Geometry: final body of the model. Coordinates: model frame, mm. A direction names the side the tool comes from. Coordinates: 2 decimals unless noted, no trailing zeros. Order: outer loops, then holes, each group sorted by start corner. A loop starts at its lowest first (then second) coordinate and runs counter-clockwise, first axis right, second up. Notation, with made-up numbers: M -38,-14 L -23,-14 A24 ccw -23,9 Z; hole C 50,-23.5 d10. An arc over 180 degrees is marked long. Use CSV: the item, a comma, the result in double quotes. Start each with the question number.
Q1. Access query for faces 1 (the face through (0, 22.5, 0)), 2 (the face through (7.277, 22.246, -7.936)). Directions: +Z, -Z, +X, -X, +Y, -Y. A direction counts if a zero-diameter tool reaches every point of the face in a straight line with its end or side. Return the directions, or none.
Q2. Ray query, probe 1 along X at (y, z) = (7.5, 6.5); probe 2 along Z at (x, y) = (7.5, 8.75); probe 3 along Z at (x, y) = (-10.5, 20.5). Return the intervals inside material, ascending.
Q3. First-contact query: P1, Ø8, axis at x = 9, y = 4, coming from the +Z side; P2, Ø8, axis at x = 12.5, z = -5, coming from the +Y side; P3, Ø3, axis at x = -4.5, y = 6, coming from the -Z side; P4, Ø2, axis at x = -8.5, y = 6.5, coming from the +Z side. Flat tips, straight axial feed; report the tip coordinate or a pass-through.
Q4. Section query C-C, the plane y = 14. Output: boundary loops of the cut face in (x, z).
Q5. Section query A-A, the plane z = 0. Output: boundary loops of the cut face in (x, y).
Q6. Section query B-B, the plane y = 4.25. Output: boundary loops of the cut face in (x, z), and give its area (3 significant figures).
from build123d import *

# Parameters (mm, degrees)
SKETCH_1_R      = 17
EXTRUDE_1_DEPTH = 8
SKETCH_2_R      = 17
EXTRUDE_2_DEPTH = 14
EXTRUDE_2_TAPER = 24
SKETCH_4_R      = 10.766798406
EXTRUDE_3_DEPTH = 0.5


with BuildPart() as part:
    # 草图1 → 凸台-拉伸1 (new body)
    with BuildSketch(Plane(origin=(0, 0, 0), x_dir=(1, 0, 0), z_dir=(0, 1, 0))):
        with Locations(Location((0, 0, 0), (0, 0, 270))):
            Circle(SKETCH_1_R)
    extrude(amount=EXTRUDE_1_DEPTH)

    # 草图2 → 凸台-拉伸2 (add)
    with BuildSketch(Plane(origin=(0, 8, 0), x_dir=(1, 0, 0), z_dir=(0, 1, 0))):
        with Locations(Location((0, 0, 0), (0, 0, 270))):
            Circle(SKETCH_2_R)
    extrude(amount=EXTRUDE_2_DEPTH, taper=EXTRUDE_2_TAPER)

    # 草图4 → 凸台-拉伸3 (add)
    with BuildSketch(Plane(origin=(0, 22, 0), x_dir=(1, 0, 0), z_dir=(0, 1, 0))):
        with Locations(Location((0, 0, 0), (0, 0, 270))):
            Circle(SKETCH_4_R)
    extrude(amount=EXTRUDE_3_DEPTH)


solid = part.part
Responses:
1,face 1,"+Z, -Z, +X, -X, +Y"
1,face 2,"+Y"
2,probe 1,"x = -15.71 to 15.71"
2,probe 2,"z = -14.88 to 14.88"
2,probe 3,"z = -4.53 to 4.53"
3,P1,"stops at z = 16.25"
3,P2,"stops at y = 22.5"
3,P3,"stops at z = -16.73"
3,P4,"stops at z = 15.26"
4,outline,"C 0,0 d28.66"
5,outline,"M -17,0 L 17,0 L 17,8 L 10.77,22 L 10.77,22.5 L -10.77,22.5 L -10.77,22 L -17,8 Z"
6,outline,"C 0,0 d34"
6,area,"908 mm²"
